Source: CAD feature listing. Evaluate the final solid. Frame: model axes, mm. Face numbers are marked on the shaded views. A direction names the side the tool comes from. Give positions to 0.01 mm unless a question says otherwise; leave off trailing zeros. Order: outer loops, then holes, each group sorted by start corner. A loop starts at its lowest first (then second) coordinate and runs counter-clockwise, first axis right, second up. Notation, with made-up numbers: (28, 26) - (48, 26) arc R11 ccw to (48, 41) - close; hole circle Ø4 at (80.5, 46). An arc over 180 degrees is marked (long way). Use CSV: the item, a comma, the result in double quotes.
Autodesk Inventor part; units mm, degrees
ref_plane "Work Plane1" through (29, 0, 0) normal (0, -1, 0) x (1, 0, 0)
ref_plane "YZ Plane" through (0, 0, 0) normal (1, 0, 0) x (0, 1, 0)
ref_plane "XZ Plane" through (0, 0, 0) normal (0, 1, 0) x (-1, 0, 0)
sketch "Sketch1" plane through (0, 0, 0) normal (0, 0, 1) x (1, 0, 0)
  line L0 (-0.19, 0) -> (12, 0)
  line L1 (12, 0) -> (12, 2.5)
  line L2 (12, 2.5) -> (2.4, 2.5)
  line L3 (2.4, 2.5) -> (1.9091, 2.5)
  line L4 (1.9091, 2.5) -> (0, 2.5)
  line L5 (0, 2.5) -> (0, 4.75)
  line L6 (0, 4.75) -> (-2.75, 4.75)
  line L7 (-2.75, 4.75) -> (-2.75, 1.7321)
  line L8 (-2.75, 1.7321) -> (-1.19, 1.7321)
  line L9 (-1.19, 1.7321) -> (-0.19, 0)
  line L10 (-5.7, 0) -> (14.95, 0)
  line L11 (0, -0.95) -> (0, 5.7)
  line L12 (2.4, 2.5) -> (0, 2.5) construction
  dimension "d1" = 9.6
  dimension "d2" = 0.4909
  dimension "d3" = 2.75
  dimension "d4" = 1.56
  dimension "d5" = 60
  dimension "d6" = 5
  dimension "d7" = 5
  dimension "d8" = 3.4641
  dimension "d9" = 9.5
  dimension "d26" = 12
revolve "Body" add sketch "Sketch1" angle 360 about axis through (-0.19, 0, 0) along (1, 0, 0)
sketch "Sketch2" plane through (-2.75, 0, 0) normal (-1, 0, 0) x (0, 0, 1)
  circle A0 centre (0, 0) radius 1.7321
  line L0 (0, -6.65) -> (0, 6.65)
  line L1 (-6.65, 0) -> (6.65, 0)
  line L2 (1.7321, 0) -> (0.866, -1.5)
  line L3 (0.866, -1.5) -> (-0.866, -1.5)
  line L4 (-0.866, -1.5) -> (-1.7321, 0)
  line L5 (-1.7321, 0) -> (-0.866, 1.5)
  line L6 (-0.866, 1.5) -> (0.866, 1.5)
  line L7 (0.866, 1.5) -> (1.7321, 0)
extrude "Slot" add sketch "Sketch2" against normal up to next contours L7 A0 | A0 L2 | L6 L0 A0 | A0 L0 L3 | L0 L6 A0 | A0 L3 L0 | L4 A0 | A0 L5
fillet "Fillet1" radius 2.37 1 edges at (-2.75, -4.75, 0)
thread "Thread"
chamfer "Chamfer1" distance 0.4908 distance2 0.4908 1 edges at (12, -2.5, 0) measured on face at (12, -0.7741, -0.6858)
ref_plane "Work Plane1" through (29, 0, 0) normal (0, -1, 0) x (1, 0, 0)
fillet "Fillet2" radius 0.45 1 edges at (0, -2.5, 0)
equation "\"d1\" = GEL"
equation "\"d3\" = KOH"
equation "\"d4\" = INTI"
equation "\"d6\" = GD"
equation "\"d7\" = BDM"
equation "\"d8\" = 1.1547 * SW"
equation "\"d9\" = KOD"
equation "\"d26\" = NLG"
equation "\"d30\" = R"
equation "\"d17\" = RR"
equation "\"d13\" = GEL"
equation "\"d15\" = -0.5 * SPD + 0.5 * GD"
equation "\"d16\" = GUL"
equation "\"GD\" = NND"
equation "\"NLG\" = 12"
equation "\"GEL\" = 9.6"
equation "\"KOD\" = 9.5"
equation "\"KOH\" = 2.75"
equation "\"INTI\" = 1.56"
equation "\"GAL\" = 0.61345 * PTC"
equation "\"GUL\" = 0.61345 * PTC"
equation "\"BDM\" = NND"
equation "\"SW\" = 3"
equation "\"RR\" = 2.37"
equation "\"SPD\" = NND - 1.2269 * PTC"
equation "\"R\" = 0.45"
equation "\"TOA\" = 30deg"
equation "\"GD1\" = THREADDIA - 1.2269 * PTC"
equation "\"THREADDIA\" = 5"
equation "\"PTC\" = 0.8"
equation "\"NND\" = 5"
equation "\"KOH1\" = 0.38"
equation "\"E0\" = 3.443"
properties part number "ISO 7380-1 - M5 x 12" material "Steel"
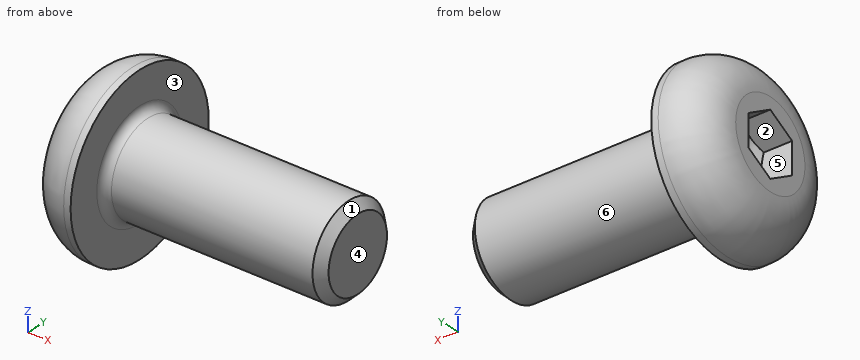
Item 1: Material intervals for line 1 (Y direction, x = 10, z = -0.75); line 2 (Y direction, x = -1.25, z = 1.5); line 3 (Y direction, x = 4, z = 2), sorted ascending. Write a range as from..to.
Filled in:
line 1,"y = -2.38..2.38"
line 2,"y = -4.33..-0.4, 0.4..4.33"
line 3,"y = -1.5..1.5"
Item 2: Set-up query: the marked faces 4, 5 and 6. Return all of +Z, -Z, +X, -X, +Y, -Y with unobstructed straight access to the full face (end or side cutting, diameter ignored); none if empty.
Filled in:
face 4,"+Z, -Z, +X, +Y, -Y"
face 5,"-X"
face 6,"+X"
Item 3: Section A-A on x = 8.25. Return the cut outline in (y, z), then the cut area to 3 significant figures.
Filled in:
outline,"circle Ø5 at (0, 0)"
area,"19.6 mm2"
Item 4: Mould query, pull axis Z, two halves, no side actions, for the marked faces 1, 2 and 3. Classes: released by +Z, released by -Z, zero draft, split by the parting line, or undercut.
Filled in:
face 1,"split by the parting line"
face 2,"undercut"
face 3,"zero draft"
Item 5: First-contact query: pin 1 (4 mm diameter, centred on x = 0, y = -3.5, fed in from -Z); pin 2 (5 mm diameter, centred on x = 4, z = 1.5, fed in from -Y); pin 3 (1.4 mm diameter, centred on x = -2, z = 0, fed in from +Y). Flat tips, straight axial feed; report the tip coordinate or a pass-through.
Filled in:
pin 1,"stops at z = -4.51"
pin 2,"stops at y = -2.5"
pin 3,"stops at y = 4.56"
